For this review, take the finished solid that the model builds, in its own axes (mm). Face numbers are marked on the shaded views. A direction names the side the tool comes from. Give positions to 0.01 mm unless a question says otherwise; leave off trailing zeros. Loops run counter-clockwise (first coordinate to the right, second up) from the corner with the lowest first, then second, coordinate; pieces in that order, holes last. Notation, with made-up numbers: (-7, 82.25) -> (12, 82.25) arc R18 cw to (12, 88.25) -> close; hole circle Ø3 at (9.25, 11). An arc over 180 degrees is marked (long way). Write each question's results on one line, items separated by ' | '. Start each with the question number.
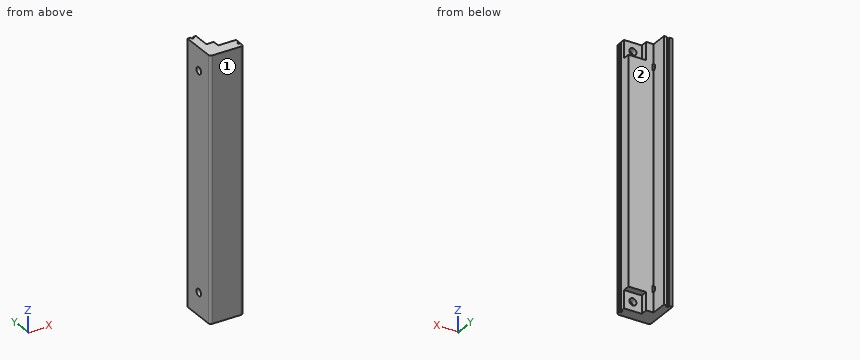
Autodesk Inventor part; units mm, degrees
ref_plane "YZ Plane" through (0, 0, 0) normal (1, 0, 0) x (0, 1, 0)
ref_plane "XZ Plane" through (0, 0, 0) normal (0, 1, 0) x (-1, 0, 0)
ref_plane "XY Plane" through (0, 0, 0) normal (0, 0, 1) x (1, 0, 0)
sketch "Sketch1" plane through (0, 0, 0) normal (0, 1, 0) x (-1, 0, 0)
  line L0 (18.1065, 110) -> (-18.1065, 110)
  line L1 (-18.1065, 110) -> (-18.1065, -110)
  line L2 (-18.1065, -110) -> (18.1065, -110)
  line L3 (18.1065, -110) -> (18.1065, 110)
  point P0 (0, 0)
  point P1 (0, 110)
  point P2 (18.1065, 0)
  dimension "d0" = 220
  dimension "d1" = 36.213
extrude "Extrusion1" add sketch "Sketch1" along normal blind 15
sketch "Sketch2" plane through (0, 15, 0) normal (0, 1, 0) x (1, 0, 0)
  line L0 (-18.1065, 110) -> (-18.1065, -110)
  line L1 (18.1065, 110) -> (-18.1065, 110)
  line L2 (-18.1065, -110) -> (-3.1065, -110)
  line L3 (-3.1065, -110) -> (-3.1065, 110)
  line L4 (-3.1065, 110) -> (-18.1065, 110)
  line L5 (-18.1065, 110) -> (-18.1065, -110)
  point P0 (0, 0)
  dimension "d4" = 15
extrude "Extrusion2" add sketch "Sketch2" along normal blind 14
sketch "Sketch3" plane through (0, 15, 0) normal (0, 1, 0) x (1, 0, 0)
  line L0 (-18.1065, -110) -> (18.1065, -110)
  line L1 (18.1065, -110) -> (3.1065, -110)
  line L2 (3.1065, -110) -> (3.1065, -95)
  line L3 (3.1065, -95) -> (18.1065, -95)
  line L4 (18.1065, -95) -> (18.1065, -110)
  point P0 (0, 0)
  dimension "d7" = 15
  dimension "d8" = 15
extrude "Extrusion3" cut sketch "Sketch3" against normal blind 6
mirror "Mirror1" about plane through (0, 0, 0) normal (0, 0, 1) of "Extrusion3"
sketch "Sketch4" plane through (0, 9, 0) normal (0, 1, 0) x (1, 0, 0)
  line L0 (18.1065, -95) -> (18.1065, -110)
  line L1 (18.1065, -110) -> (3.1065, -110)
  point P0 (0, 0)
  point P1 (10.6065, -102.5)
  point P2 (18.1065, -102.5)
  dimension "d11" = 7.5
  dimension "d12" = 7.5
hole "Hole1" at (10.6065, 9, 102.5) direction (0, -1, 0) diameter 6 depth 5
mirror "Mirror2" about plane through (0, 0, 0) normal (0, 0, 1) of "Hole1"
sketch "Sketch5" plane through (-18.1065, 0, 110) normal (0, 0, 1) x (1, 0, 0)
  point P0 (18.1065, 0)
move faces "Move2" translate (7.929, 0, 0) faces at (-18.1065, 9.6667, -36.6667)
move faces "Move3" translate (0, -1, 0) faces at (8.6785, 0, 36.6667)
sketch "Sketch6" plane through (18.1065, 9, 95) normal (1, 0, 0) x (0, 0, -1)
  line L0 (205, -10) -> (205, 0)
  line L1 (-15, -10) -> (-15, 0)
  line L2 (205, -5.9) -> (-15, -5.9)
  line L3 (205, -5) -> (-15, -5)
  line L4 (205, -4.1) -> (-15, -4.1)
  line L5 (205, -4.1) -> (205, -5.9)
  line L6 (205, -10) -> (205, 20)
  line L7 (-15, -4.1) -> (-15, -5.9)
  point P0 (95, -9)
  dimension "d29" = 1.8
extrude "Extrusion4" cut sketch "Sketch6" against normal blind 1.6
sketch "Sketch7" plane through (0, 29, 0) normal (0, 1, 0) x (1, 0, 0)
  line L0 (-6.642, 113.6406) -> (-6.642, -120.3961) construction
  line L1 (-3.1065, 110) -> (-10.1775, 110)
  line L2 (18.1065, 110) -> (-10.1775, 110)
  line L3 (-5.742, 110) -> (-5.742, -110)
  line L4 (-10.1775, -110) -> (-3.1065, -110)
  line L5 (-7.542, 110) -> (-7.542, -110)
  line L6 (-5.742, 110) -> (-7.542, 110)
  line L7 (-5.742, -110) -> (-7.542, -110)
  point P0 (0, 0)
  point P1 (-6.642, 110)
  point P2 (-7.542, 110)
  point P3 (-7.542, -110)
  point P4 (-5.742, 110)
  dimension "d35" = 1.8
extrude "Extrusion5" cut sketch "Sketch7" against normal blind 1.8
sketch "Sketch16" plane through (-10.1775, 29, -110) normal (-1, 0, 0) x (0, 0, 1)
  line L0 (0, -30) -> (0, 0)
  line L1 (220, -30) -> (220, 0)
  line L2 (0, 0) -> (220, 0)
  point P0 (110, -29)
  point P1 (19.142, -15)
  point P2 (200.858, -15)
  dimension "d75" = 181.716
  dimension "d76" = 220
  dimension "d77" = 19.142
  dimension "d78" = 30
  dimension "d79" = 15
hole "Hole6" at (-10.1775, 14, 90.858) at (-10.1775, 14, -90.858) direction (1, 0, 0) diameter 6 depth 8
fillet "Fillet1" radius 2 1 edges at (-10.1775, -1, 0)
fillet "Fillet2" radius 2 1 edges at (18.1065, -1, 0)
equation "\"d8\" = d7"
properties part number "top_edge" material "ABS Plastic"
1. We need section A-A (x = 5.5). Write out the cut boundary in (y, z).
2. We need section D-D (z = 102.5). Write out the cut boundary in (x, y).
3. We need section C-C (y = 24.5). Write out the cut boundary in (x, z), plus the area to 3 significant figures.
4. Machinability: for the marked faces 1 and 2, which of the approach directions +Z, -Z, +X, -X, +Y, -Y give a long, thin tool a straight path to every point of the face, cutting with its end or side? Answer none if there is none.
5. Wall thickness on L1, parallel to Z at x = -7.25, y = 14; L2, parallel to X at y = 27.5, z = -66.5; L3, parallel to Y at x = 7.5, z = 13.5: over which ranges is each line inside the solid? List them lowest first.
6. For pin 1 Ø5 at (x, z) = (10.61, 102.5) entering from +Y; pin 2 Ø3 at (x, y) = (9, 13.5) entering from -Z; pin 3 Ø0.9 at (x, z) = (-6.5, -41.5) entering from +Y, all flat-tipped, find the tip position at first contact; note any pin that passes through.
7. We need section B-B (z = -53). Write out the cut boundary in (x, y), plus the area to 3 significant figures.
Response:
1) outline: (-1, -110) -> (9, -110) -> (9, -95) -> (15, -95) -> (15, 95) -> (9, 95) -> (9, 110) -> (-1, 110) -> close
2) outline: (-10.18, 1) arc R2 ccw to (-8.18, -1) -> (16.11, -1) arc R2 ccw to (18.11, 1) -> (18.11, 3.1) -> (16.51, 3.1) -> (16.51, 4.9) -> (18.11, 4.9) -> (18.11, 9) -> (13.61, 9) -> (13.61, 4) -> (7.61, 4) -> (7.61, 9) -> (3.11, 9) -> (3.11, 15) -> (-3.11, 15) -> (-3.11, 29) -> (-5.74, 29) -> (-5.74, 27.2) -> (-7.54, 27.2) -> (-7.54, 29) -> (-10.18, 29) -> close
3) outline: (-10.18, -110) -> (-3.11, -110) -> (-3.11, 110) -> (-10.18, 110) -> close | area: 1,560 mm2
4) face 1: +Z, -Z, +X, -X, -Y | face 2: +Z, -Z, +X, +Y
5) L1: z = -110 to -93.86, -87.86 to 87.86, 93.86 to 110 | L2: x = -10.18 to -7.54, -5.74 to -3.11 | L3: y = -1 to 15
6) pin 1: stops at y = 4 | pin 2: stops at z = -95 | pin 3: stops at y = 27.2
7) outline: (-10.18, 1) arc R2 ccw to (-8.18, -1) -> (16.11, -1) arc R2 ccw to (18.11, 1) -> (18.11, 3.1) -> (16.51, 3.1) -> (16.51, 4.9) -> (18.11, 4.9) -> (18.11, 15) -> (-3.11, 15) -> (-3.11, 29) -> (-5.74, 29) -> (-5.74, 27.2) -> (-7.54, 27.2) -> (-7.54, 29) -> (-10.18, 29) -> close | area: 544 mm2
